Work out the finished part from the listing and answer in its coordinate system (mm). Face numbers are marked on the shaded views. A direction names the side the tool comes from. Give positions to 0.01 mm unless a question says otherwise; leave off trailing zeros. Loops run counter-clockwise (first coordinate to the right, second up) from the corner with the lowest first, then second, coordinate; pieces in that order, holes last. Notation, with made-up numbers: M 60,79.5 L 78,79.5 A25 ccw 78,109.5 Z; hole C -35,47.5 d6. An arc over 180 degrees is marked long. Write item = value, one per line. Start each with the question number.
1. Flat-ended cylindrical pins translate along their axes: pin 1 Ø5.5 at (y, z) = (2.5, 156) entering from +X; pin 2 Ø1.5 at (y, z) = (1.5, 154) entering from -X; pin 3 Ø4 at (y, z) = (606.5, 157) entering from +X; pin 4 Ø5.5 at (x, y) = (-160, 607) entering from -Z. Find the tip coordinate at first contact, or state that the pin passes through.
2. Section D-D on y = 144 is taken. Determine the outline of the cut face in (x, z).
3. Section A-A on x = -308 is taken. Determine the outline of the cut face in (y, z).
4. Section C-C on z = 650 is taken. Determine the outline of the cut face in (x, y), plus the area to 3 significant figures.
5. For the marked faces 4 and 5, determine the directions among +Z, -Z, +X, -X, +Y, -Y from which every point of the face is accessible in a straight line to the end or side of a thin tool.
6. Consider L1, parallel to Y at x = -64.5, z = 1027.5; L2, parallel to X at y = 535, z = 271; L3, parallel to X at y = 307.5, z = 532.5. Determine where each line is inside the solid, lowest interval first. Write a range as [from, to].
7. Section B-B on y = 572 is taken. Determine the outline of the cut face in (x, z).
8. The mould has two halves that part along Y. Classify the marked faces 1, 2 and 3: released by +Y, released by -Y, zero draft, split by the parting line, or undercut.
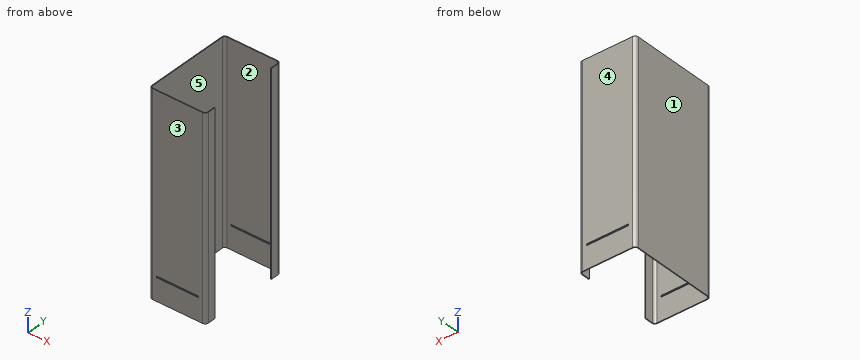
```python
from build123d import *

# Parameters (mm, degrees)
F1_DEPTH = 1341
F2_W     = 283
F2_H     = 11
F3_DEPTH = 610


with BuildPart() as f1:
    # F0 (on Top) → F1 (new body)
    with BuildSketch(Plane.XY):
        with BuildLine():
            Line((-360, 0), (-21, 0))
            ThreePointArc((-21, 0), (-6.150758, 6.150758), (0, 21))
            Line((0, 21), (0, 76.5))
            Line((0, 76.5), (-5, 76.5))
            Line((-5, 76.5), (-5, 21))
            ThreePointArc((-5, 21), (-9.686292, 9.686292), (-21, 5))
            Line((-21, 5), (-360, 5))
            ThreePointArc((-360, 5), (-371.313708, 9.686292), (-376, 21))
            Line((-376, 21), (-376, 589))
            ThreePointArc((-376, 589), (-371.313708, 600.313708), (-360, 605))
            Line((-360, 605), (-21, 605))
            ThreePointArc((-21, 605), (-9.686292, 600.313708), (-5, 589))
            Line((-5, 589), (-5, 533.5))
            Line((-5, 533.5), (0, 533.5))
            Line((0, 533.5), (0, 589))
            ThreePointArc((0, 589), (-6.150758, 603.849242), (-21, 610))
            Line((-21, 610), (-360, 610))
            ThreePointArc((-360, 610), (-374.849242, 603.849242), (-381, 589))
            Line((-381, 589), (-381, 21))
            ThreePointArc((-381, 21), (-374.849242, 6.150758), (-360, 0))
        make_face()
    extrude(amount=F1_DEPTH)

    # F2 (on face) → F3 (cut, through all)
    with BuildSketch(Plane(origin=(0, 610, 0), x_dir=(-1, 0, 0), z_dir=(0, 1, 0))):
        with Locations((190.5, 156.5)):
            Rectangle(F2_W, F2_H)
    extrude(amount=-F3_DEPTH, mode=Mode.SUBTRACT)


solid = f1.part
```
Verdict:
q1.pin_1 = -7.11
q1.pin_2 = -369.46
q1.pin_3 = -6.83
q1.pin_4 = 0
q2.outline = M -381,0 L -376,0 L -376,1341 L -381,1341 Z
q3.outline = M 0,0 L 5,0 L 5,151 L 0,151 Z; M 0,162 L 5,162 L 5,1341 L 0,1341 Z; M 605,0 L 610,0 L 610,151 L 605,151 Z; M 605,162 L 610,162 L 610,1341 L 605,1341 Z
q4.outline = M -381,21 A21 ccw -360,0 L -21,0 A21 ccw 0,21 L 0,76.5 L -5,76.5 L -5,21 A16 cw -21,5 L -360,5 A16 cw -376,21 L -376,589 A16 cw -360,605 L -21,605 A16 cw -5,589 L -5,533.5 L 0,533.5 L 0,589 A21 ccw -21,610 L -360,610 A21 ccw -381,589 Z
q4.area = 7,370 mm2
q5.face_4 = +Z, -Z, +X, -X, +Y
q5.face_5 = +Z, -Z
q6.L1 = [0, 5], [605, 610]
q6.L2 = [-381, -376], [-5, 0]
q6.L3 = [-381, -376]
q7.outline = M -381,0 L -376,0 L -376,1341 L -381,1341 Z; M -5,0 L 0,0 L 0,1341 L -5,1341 Z
q8.face_1 = zero draft
q8.face_2 = undercut
q8.face_3 = released by -Y
